For this review, take the finished solid that the model builds, in its own axes (mm). A direction names the side the tool comes from. Coordinates: 2 decimals unless noted, no trailing zeros. Loops run counter-clockwise (first coordinate to the right, second up) from the corner with the lowest first, then second, coordinate; pieces in that order, holes last. Notation, with made-up numbers: M 23.5,51.5 L 82.5,51.5 A18 cw 82.5,58.5 Z; hole C 83.25,82.25 d11. An arc over 180 degrees is marked long. Answer as a JSON object with one key per item and string values. Group by question number.
Item 1: Wall thickness on L1, parallel to Y at x = 0, z = 2.45; L2, parallel to X at y = 2, z = 4.75; L3, parallel to X at y = -19, z = 3.25: over which ranges is each line inside the solid? List them lowest first. Write a range as from..to.
Item 2: Add section C-C (y = -20). State the section outline as (x, z) points.
Item 3: Insertion check: pin 1 (2 mm diameter, centred on y = 12, z = 2.5, fed in from -X); pin 2 (1 mm diameter, centred on x = 15, z = 4, fed in from -Y); pin 3 (3 mm diameter, centred on y = 20, z = 3.5, fed in from -X). Each pin has a flat end and moves straight along its axis. Give the tip position at first contact, or say it passes through.
Item 4: Mouldability with a two-part tool opening along Y and no side actions: class faces 1 (the face through (10.9, -5.14, 2.54)), 2 (the face through (-6.2, 0.4, 0)), 3 (the face through (-17.854, 0.676, 2.465)), 4 (the face through (-22.783, -10.292, 2.465)) as +Y half, -Y half, draft (parallel to the pull), parting line (faces both ways), or undercut.
Item 5: Add section B-B (z = 4.1). State the section outline as (x, y) points.
Item 6: Add section A-A (y = 0). State the section outline as (x, z) points.
Item 7: Add section D-D (x = 0). State the section outline as (y, z) points.
Item 8: Tool access review of faces 5 (the face through (-0.488, 17.804, 2.465)), 6 (the face through (10, 10, 2)): name each direction out of +Z, -Z, +X, -X, +Y, -Y from which nothing blocks a thin tool from reaching the whole face with its end or side.
from build123d import *

# Parameters (mm, degrees)
SKIZZE1_R                       = 25
SKIZZE1_R_2                     = 6
SKIZZE1_R_3                     = 2.25
AUFSATZ_LINEAR_AUSTRAGEN1_DEPTH = 5
SKIZZE2_W                       = 24.326966906
SKIZZE2_H                       = 39.351197917
SCHNITT_LINEAR_AUSTRAGEN1_DEPTH = 5
VERRUNDUNG1_R                   = 3


with BuildPart() as part:
    # Skizze1 → Aufsatz-Linear austragen1 (new body)
    with BuildSketch(Plane.XY):
        Circle(SKIZZE1_R)
        Circle(SKIZZE1_R_2, mode=Mode.SUBTRACT)
        with Locations((0, 20)):
            Circle(SKIZZE1_R_3, mode=Mode.SUBTRACT)
        with Locations((-20, 0)):
            Circle(SKIZZE1_R_3, mode=Mode.SUBTRACT)
        with Locations((0, -20)):
            Circle(SKIZZE1_R_3, mode=Mode.SUBTRACT)
    extrude(amount=AUFSATZ_LINEAR_AUSTRAGEN1_DEPTH)

    # Skizze2 → Schnitt-Linear austragen1 (cut)
    with BuildSketch(Plane(origin=(0, 0, 0), x_dir=(-1, 0, 0), z_dir=(0, 0, -1))):
        with Locations((-22.163483453, 13.675598959)):
            Rectangle(SKIZZE2_W, SKIZZE2_H)
    extrude(amount=-SCHNITT_LINEAR_AUSTRAGEN1_DEPTH, mode=Mode.SUBTRACT)

    # Verrundung1
    verrundung1_edges = [part.edges().sort_by_distance(p)[0] for p in [
        (10, -6, 2.5),
    ]]
    fillet(verrundung1_edges, radius=VERRUNDUNG1_R)


solid = part.part
From the geometry:
{
 "1": {"L1": "y = -25..-22.25, -17.75..-6, 6..17.75, 22.25..25", "L2": "x = -24.92..-21.03, -18.97..-5.66, 5.66..10", "L3": "x = -16.25..-2.02, 2.02..16.25"},
 "2": {"outline": "M -15,0 L -2.25,0 L -2.25,5 L -15,5 Z; M 2.25,0 L 15,0 L 15,5 L 2.25,5 Z"},
 "3": {"pin 1": "stops at x = -22.45", "pin 2": "stops at y = -20.37", "pin 3": "stops at x = -16.82"},
 "4": {"face 1": "+Y half", "face 2": "draft", "face 3": "undercut", "face 4": "parting line"},
 "5": {"outline": "M 10,-3 L 10,22.91 A25 ccw long 24.27,-6 L 13,-6 A3 cw Z; hole C -20,0 d4.5; hole C 0,0 d12; hole C 0,-20 d4.5; hole C 0,20 d4.5"},
 "6": {"outline": "M -25,0 L -22.25,0 L -22.25,5 L -25,5 Z; M -17.75,0 L -6,0 L -6,5 L -17.75,5 Z; M 6,0 L 10,0 L 10,5 L 6,5 Z"},
 "7": {"outline": "M -25,0 L -22.25,0 L -22.25,5 L -25,5 Z; M -17.75,0 L -6,0 L -6,5 L -17.75,5 Z; M 6,0 L 17.75,0 L 17.75,5 L 6,5 Z; M 22.25,0 L 25,0 L 25,5 L 22.25,5 Z"},
 "8": {"face 5": "+Z, -Z", "face 6": "+Z, -Z, +X, +Y"}
}
